The listing builds one solid part. Answer for the finished solid, in the listing's coordinates (mm). A direction names the side the tool comes from. Give positions to 0.01 mm unless a question says otherwise; leave off trailing zeros. Loops run counter-clockwise (first coordinate to the right, second up) from the corner with the lowest first, then second, coordinate; pieces in that order, holes last. Notation, with made-up numbers: M 51.25,34 L 60.25,34 A20 ccw 60.25,57 Z; hole C 29,8 d9. An arc over 180 degrees is marked long. One line per item, written item: value. Start each with the question number.
Q1. A cutting plane is placed at C-C, the plane x = -1338. Determine the outline of the cut face in (y, z), and give its area (4 significant figures).
Q2. A cutting plane is placed at A-A, the plane z = 352. Determine the outline of the cut face in (x, y), and give its area (3 significant figures).
Q3. The mould has two halves that part along X. Classify faces 4 (the flat face through (-825, 301, 393.7)), 5 (the flat face through (76.2, 301, 220)), 6 (the flat face through (57.15, 310, 210)): +X half, -X half, draft (parallel to the pull), parting line (faces both ways), or undercut.
Q4. For faces 1 (the flat face through (63, 247, 50.8)), 2 (the flat face through (-842, 609.6, 390)), 3 (the flat face through (-1162.05, 310, 185)), determine the directions among +Z, -Z, +X, -X, +Y, -Y from which every point of the face is accessible in a straight line to the end or side of a thin tool.
Q5. A cutting plane is placed at B-B, the plane y = 247. Determine the outline of the cut face in (x, z).
Q6. Flat-ended cylindrical pins translate along their axes: pin 1 (21 mm diameter, centred on x = -1743, z = 95, fed in from +Y) (3 decimals); pin 2 (3 mm diameter, centred on x = -1408.5, z = 231.5, fed in from +Y); pin 3 (15 mm diameter, centred on y = 12.5, z = 35.5, fed in from +X). Find the tip coordinate at first contact, or state that the pin passes through.
Q7. Consider L1, parallel to X at y = 177.5, z = 174.5; L2, parallel to Z at x = -1557, y = 202.5. Determine where each line is inside the solid, lowest interval first.
from build123d import *

# Parameters (mm, degrees)
F0_W     = 19.05
F0_H     = 374.65
F0_H_2   = 323.85
F1_DEPTH = 609.6
F0_W_2   = 571.5
F0_W_3   = 590.55
F2_DEPTH = 19.05
F3_W     = 73.025
F3_H     = 171.45
F4_DEPTH = 1828.8


with BuildPart() as f1:
    # F0 (on Front) → F1 (new body)
    with BuildSketch(Plane.XZ):
        with Locations((-1743.075, 187.325)):
            Rectangle(F0_W, F0_H)
        Polygon((-552.45, 374.65), (-533.4, 374.65), (57.15, 374.65), (76.2, 374.65), (76.2, 393.7), (-1752.6, 393.7), (-1752.6, 374.65), (-1733.55, 374.65), (-1162.05, 374.65), (-1143, 374.65), align=None)
        with Locations((-1152.525, 187.325)):
            Rectangle(F0_W, F0_H)
        with Locations((-542.925, 187.325)):
            Rectangle(F0_W, F0_H)
        with Locations((66.675, 212.725)):
            Rectangle(F0_W, F0_H_2)
    extrude(amount=-F1_DEPTH)

    # F0 (on Front) → F2 (join)
    with BuildSketch(Plane.XZ):
        with Locations((-1743.075, 187.325)):
            Rectangle(F0_W, F0_H)
        with Locations((-1447.8, 187.325)):
            Rectangle(F0_W_2, F0_H)
        Polygon((-552.45, 374.65), (-533.4, 374.65), (57.15, 374.65), (76.2, 374.65), (76.2, 393.7), (-1752.6, 393.7), (-1752.6, 374.65), (-1733.55, 374.65), (-1162.05, 374.65), (-1143, 374.65), align=None)
        with Locations((-847.725, 187.325)):
            Rectangle(F0_W_3, F0_H)
        with Locations((-542.925, 187.325)):
            Rectangle(F0_W, F0_H)
        Polygon((-533.4, 0), (0, 0), (0, 50.8), (57.15, 50.8), (57.15, 374.65), (-533.4, 374.65), align=None)
        with Locations((66.675, 212.725)):
            Rectangle(F0_W, F0_H_2)
    extrude(amount=-F2_DEPTH)

    # F3 (on face) → F4 (cut, through all)
    with BuildSketch(Plane(origin=(-1752.6, 0, 0), x_dir=(0, -1, 0), z_dir=(-1, 0, 0))):
        with Locations((-573.0875, 85.725)):
            Rectangle(F3_W, F3_H)
    extrude(amount=-F4_DEPTH, mode=Mode.SUBTRACT)


solid = f1.part
Answer block:
1. outline: M 0,0 L 19.05,0 L 19.05,374.65 L 609.6,374.65 L 609.6,393.7 L 0,393.7 Z
1. area: 18,750 mm^2
2. outline: M -1752.6,0 L 76.2,0 L 76.2,609.6 L 57.15,609.6 L 57.15,19.05 L -533.4,19.05 L -533.4,609.6 L -552.45,609.6 L -552.45,19.05 L -1143,19.05 L -1143,609.6 L -1162.05,609.6 L -1162.05,19.05 L -1733.55,19.05 L -1733.55,609.6 L -1752.6,609.6 Z
2. area: 79,800 mm^2
3. face 4: draft
3. face 5: +X half
3. face 6: undercut
4. face 1: -Z, +X, +Y, -Y
4. face 2: +Z, -Z, +X, -X, +Y
4. face 3: -Z, +Y
5. outline: M -1752.6,0 L -1733.55,0 L -1733.55,374.65 L -1162.05,374.65 L -1162.05,0 L -1143,0 L -1143,374.65 L -552.45,374.65 L -552.45,0 L -533.4,0 L -533.4,374.65 L 57.15,374.65 L 57.15,50.8 L 76.2,50.8 L 76.2,393.7 L -1752.6,393.7 Z
6. pin 1: y = 536.575
6. pin 2: y = 19.05
6. pin 3: x = 0
7. L1: -1752.6 to -1733.55, -1162.05 to -1143, -552.45 to -533.4, 57.15 to 76.2
7. L2: 374.65 to 393.7
